The drawing under review shows one solid part. Ordinate dimensions are in mm from its lowest x, y, z. A direction names the side the tool comes from. Coordinates: 2 decimals unless noted, no trailing zeros. Write each loop counter-clockwise with the first axis right and the second up, starting at its lowest first coordinate (ties: lowest second). Pieces come first, ordered by that corner, then holes.
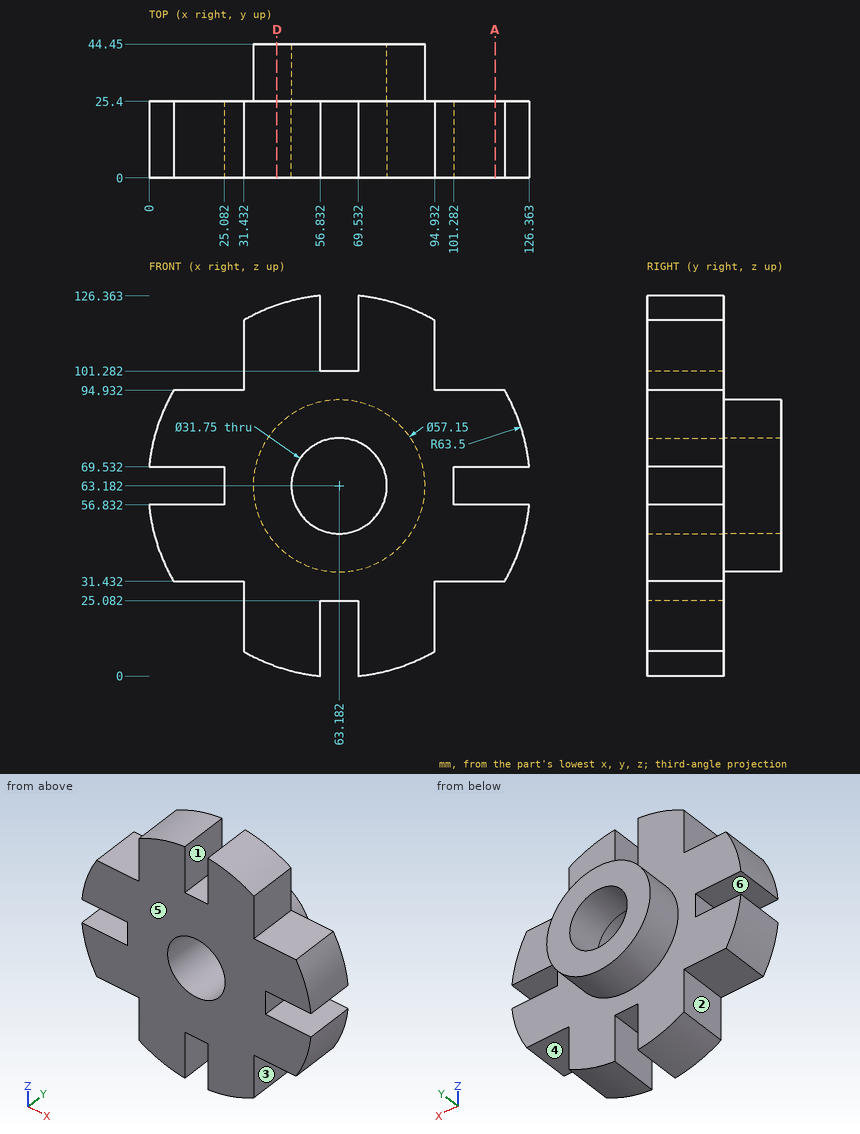
Q1. Tool access review of the marked faces 1, 2 and 3: name each direction out of +Z, -Z, +X, -X, +Y, -Y from which nothing blocks a thin tool from reaching the whole face with its end or side.
Ans:
face 1: +Z, +Y, -Y
face 2: -Z, -X, +Y, -Y
face 3: -Z, +X, +Y, -Y
Q2. Add section D-D (x = 42.5). State the section outline as (y, z) points, then the cut area to 3 significant figures.
Ans:
outline: (0, 3.14) - (25.4, 3.14) - (25.4, 43.46) - (44.45, 43.46) - (44.45, 82.9) - (25.4, 82.9) - (25.4, 123.22) - (0, 123.22) - close
area: 3,800 mm2
Q3. Draft analysis for pull direction Z (two halves, no side actions). For the marked faces 4, 5 and 6, state which applies: +Z half, -Z half, draft (parallel to the pull), parting line (faces both ways), or undercut.
Ans:
face 4: -Z half
face 5: draft
face 6: undercut
Q4. Add section A-A (x = 115). State the section outline as (y, z) points, then the cut area to 3 significant figures.
Ans:
outline: (0, 31.43) - (25.4, 31.43) - (25.4, 56.83) - (0, 56.83) - close; (0, 69.53) - (25.4, 69.53) - (25.4, 94.93) - (0, 94.93) - close
area: 1,290 mm2
Q5. Clearance check with flat-ended pins moving along their axes: pin 1 Ø3 at (x, z) = (55.5, 19) entering from +Y; pin 2 Ø11.5 at (y, z) = (11.5, 21) entering from -X; pin 3 Ø10 at (x, y) = (65.5, 12) entering from +Z; pin 4 Ø12 at (x, y) = (19, 32.5) entering from -Z. State where each tip first meets the part, or that it passes through.
Ans:
pin 1: stops at y = 25.4
pin 2: stops at x = 31.43
pin 3: stops at z = 126.36
pin 4: passes through
Q6. For probe 1 along X at (y, z) = (16.5, 102); probe 2 along Z at (x, y) = (62.5, 16.5), list the stretches that pass through material, from the lowest coordinate up.
Ans:
probe 1: x = 31.43 to 56.83, 69.53 to 94.93
probe 2: z = 25.08 to 47.32, 79.04 to 101.28
